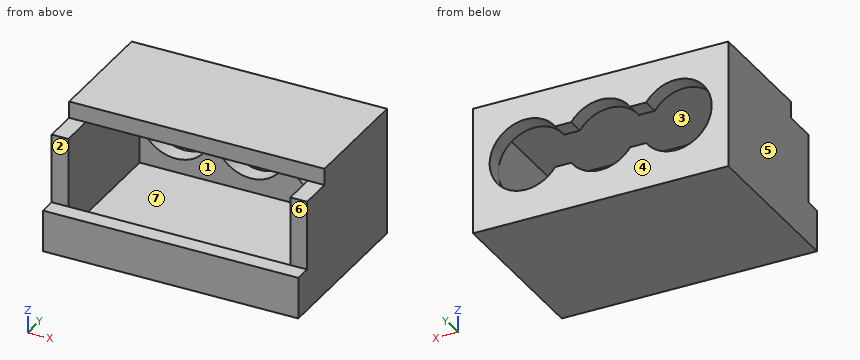
```python
from build123d import *

# Parameters (mm, degrees)
SKETCH_W        = 18.4
SKETCH_H        = 11
PAD_DEPTH       = 8
SKETCH002_R     = 2.6
POCKET_DEPTH    = 10
SKETCH003_W     = 16
SKETCH003_H     = 9.8
POCKET001_DEPTH = 6.8
SKETCH004_W     = 10.8
SKETCH004_H     = 3
POCKET002_DEPTH = 5
SKETCH005_W     = 18.4
SKETCH005_H     = 3
PAD001_DEPTH    = 1.2
SKETCH006_W     = 18.4
SKETCH006_H     = 8.6
PAD002_DEPTH    = 1.2


with BuildPart() as part:
    # Sketch → Pad (new body)
    with BuildSketch(Plane.XY):
        Rectangle(SKETCH_W, SKETCH_H)
    extrude(amount=PAD_DEPTH)

    # Sketch002 (on Face3 of Pad) → Pocket (cut)
    with BuildSketch(Plane(origin=(0, 5.5, 0), x_dir=(-1, 0, 0), z_dir=(0, 1, 0))):
        with Locations((-5.4, 4.8)):
            Circle(SKETCH002_R)
        with Locations((0, 4.8)):
            Circle(SKETCH002_R)
        with Locations((5.4, 4.8)):
            Circle(SKETCH002_R)
    extrude(amount=-POCKET_DEPTH, mode=Mode.SUBTRACT)

    # Sketch003 (on Face5 of Pocket) → Pocket001 (cut)
    with BuildSketch(Plane.XY.offset(8)):
        with Locations((0, -0.6)):
            Rectangle(SKETCH003_W, SKETCH003_H)
    extrude(amount=-POCKET001_DEPTH, mode=Mode.SUBTRACT)

    # Sketch004 (on Face9 of Pocket001) → Pocket002 (cut)
    with BuildSketch(Plane(origin=(0, 5.5, 0), x_dir=(-1, 0, 0), z_dir=(0, 1, 0))):
        with Locations((0, 4.8)):
            Rectangle(SKETCH004_W, SKETCH004_H)
    extrude(amount=-POCKET002_DEPTH, mode=Mode.SUBTRACT)

    # Sketch005 (on Face1 of Pocket002) → Pad001 (join)
    with BuildSketch(Plane.XZ.offset(5.5)):
        with Locations((0, 1.5)):
            Rectangle(SKETCH005_W, SKETCH005_H)
    extrude(amount=PAD001_DEPTH)

    # Sketch006 (on Face4 of Pad001) → Pad002 (join)
    with BuildSketch(Plane.XY.offset(8)):
        with Locations((0, 1.2)):
            Rectangle(SKETCH006_W, SKETCH006_H)
    extrude(amount=PAD002_DEPTH)


solid = part.part
```
Part model, mm, in its own coordinate system. Face numbers are marked on the shaded views. A direction names the side the tool comes from. Coordinates: 2 decimals unless noted, no trailing zeros. Order: outer loops, then holes, each group sorted by start corner. A loop starts at its lowest first (then second) coordinate and runs counter-clockwise, first axis right, second up. Notation, with made-up numbers: (-5.75, -25.75) - (8.25, -25.75) arc R23 ccw to (8.25, -9.75) - close; hole circle Ø10 at (23.25, 79). An arc over 180 degrees is marked (long way). Return JSON: item names as keys, results as strings. Group by question number.
Item 1: Which spindle directions (+Z, -Z, +X, -X, +Y, -Y) get a long thin tool onto all of the face, cutting with end or side? Do the marked faces 1, 2 and 3. Say none if no direction does.
Item 2: Pull direction Y, two halves, no side cores. Call the marked faces 4, 5, 6 and 7: pulls with the +Y half, pulls with the -Y half, needs draft (parallel to the pull), parting line crosses it, or undercut.
Item 3: Cut at A-A (x = -2.5). List the corners of the cut face in (y, z).
Item 4: Drill centre lines: probe 1 along X at (y, z) = (5.1, 4.8); probe 2 along Z at (x, y) = (-5.4, 4.8); probe 3 along Z at (x, y) = (6.75, 1.5). Where is each one in solid material? Low to high. Write a range as from..to.
Item 5: Cut at C-C (x = 6). List the corners of the cut face in (y, z), plus the area to 3 significant figures.
Item 6: Cut at B-B (y = 4). List the corners of the cut face in (x, z), plus the area to 3 significant figures.
Item 7: Pin check, flat tips, straight feed: pin 1 (4 mm diameter, centred on x = 0.5, z = 3.5, fed in from -Y); pin 2 (2.5 mm diameter, centred on x = -1.5, z = 7, fed in from -Y); pin 3 (1.3 mm diameter, centred on x = 8.5, y = -4.5, fed in from +Z). Stop position of each tip, or through.
Check values:
{
 "1": {"face 1": "none", "face 2": "+Z, +X, -X, -Y", "face 3": "-Y"},
 "2": {"face 4": "pulls with the +Y half", "face 5": "needs draft", "face 6": "pulls with the -Y half", "face 7": "undercut"},
 "3": {"outline": "(-6.7, 0) - (5.5, 0) - (5.5, 3.3) - (4.3, 3.3) - (4.3, 1.2) - (-5.5, 1.2) - (-5.5, 3) - (-6.7, 3) - close; (-3.1, 8) - (4.3, 8) - (4.3, 6.3) - (5.5, 6.3) - (5.5, 9.2) - (-3.1, 9.2) - close"},
 "4": {"probe 1": "x = -9.2..-8, 8..9.2", "probe 2": "z = 0..2.2, 7.4..9.2", "probe 3": "z = 0..1.2, 8..9.2"},
 "5": {"outline": "(-6.7, 0) - (5.5, 0) - (5.5, 2.27) - (4.3, 2.27) - (4.3, 1.2) - (-5.5, 1.2) - (-5.5, 3) - (-6.7, 3) - close; (-3.1, 8) - (4.3, 8) - (4.3, 7.33) - (5.5, 7.33) - (5.5, 9.2) - (-3.1, 9.2) - close", "area": "29.2 mm2"},
 "6": {"outline": "(-9.2, 0) - (9.2, 0) - (9.2, 9.2) - (-9.2, 9.2) - close; hole (-8, 1.2) - (8, 1.2) - (8, 8) - (-8, 8) - close", "area": "60.5 mm2"},
 "7": {"pin 1": "stops at y = -6.7", "pin 2": "stops at y = -3.1", "pin 3": "stops at z = 8"}
}
